Autodesk Inventor part; units mm, degrees
ref_plane "YZ Plane" through (0, 0, 0) normal (1, 0, 0) x (0, 1, 0)
ref_plane "XZ Plane" through (0, 0, 0) normal (0, 1, 0) x (-1, 0, 0)
ref_plane "XY Plane" through (0, 0, 0) normal (0, 0, 1) x (1, 0, 0)
sketch "Sketch1" plane through (0, 0, 0) normal (0, 0, 1) x (1, 0, 0)
  line L0 (-75, 42.5) -> (75, 42.5)
  line L1 (75, 42.5) -> (75, -107.5)
  line L2 (75, -107.5) -> (-75, -107.5)
  line L3 (-75, -107.5) -> (-75, 42.5)
  point P0 (0, 0)
  dimension "d0" = 150
  dimension "d1" = 75
  dimension "d2" = 150
  dimension "d85" = 42.5
extrude "baseExtrusion" add sketch "Sketch1" along normal blind 10
sketch "Sketch3" plane through (0, 0, 10) normal (0, 0, 1) x (1, 0, 0)
  circle A0 centre (0, -22.5) radius 21.25
  line L0 (-75, -107.5) -> (75, -107.5)
  line L1 (-75, 42.5) -> (-75, -107.5)
  line L2 (75, 42.5) -> (-75, 42.5)
  dimension "d16" = 42.5
  dimension "d68" = 75
  dimension "d84" = 65
extrude "objectiveExtrusion" cut sketch "Sketch3" against normal through all
sketch "Sketch5" plane through (0, 0, 10) normal (0, 0, 1) x (1, 0, 0)
  line L0 (30, 15) -> (75, 15)
  line L1 (75, 15) -> (75, 0)
  line L2 (75, 0) -> (30, 0)
  line L3 (22.5, 7.5) -> (22.5, 7.5)
  line L4 (75, -107.5) -> (75, 42.5)
  arc A0 (30, 15) -> (22.5, 7.5) centre (30, 7.5) ccw
  arc A1 (22.5, 7.5) -> (30, 0) centre (30, 7.5) ccw
  circle A2 centre (0, -22.5) radius 21.25
  point P0 (0, 0)
  point P1 (22.5, 15)
  dimension "d34" = 15
  dimension "d35" = 7.5
  dimension "d54" = 30
  dimension "d67" = 30
extrude "cageRodBase1" cut sketch "Sketch5" against normal through all contours L0 L1 L2 A1 A0
mirror "cageRodBase2" about plane through (0, 0, 0) normal (1, 0, 0) of "cageRodBase1"
pattern_linear "cageRodBase34" count 2 spacing 60 along (0, -1, 0) of "cageRodBase1", "cageRodBase2"
sketch "Sketch8" plane through (0, 0, 0) normal (0, 0, -1) x (-1, 0, 0)
  line L0 (75, 0) -> (75, -45)
  line L1 (75, 15) -> (75, 42.5)
  circle A0 centre (0, -22.5) radius 21.25
  point P0 (0, 0)
  point P1 (0, 5)
  point P2 (-23.8157, -36.25)
  point P3 (23.8157, -36.25)
  dimension "d71" = 75
  dimension "d72" = 27.5
  dimension "d75" = 360
hole "objectiveHolderMountingHoles" at (-23.8157, -36.25, 0) at (23.8157, -36.25, 0) at (0, 5, 0) direction (0, 0, 1) diameter 3.242 end through all
sketch "Sketch9" plane through (0, 0, 0) normal (0, 0, -1) x (-1, 0, 0)
  line L0 (75, -60) -> (30, -60)
  line L1 (30, -45) -> (75, -45)
  arc A0 (30, -45) -> (30, -60) centre (30, -52.5) ccw
  point P0 (0, 0)
  point P1 (60, -70)
  point P2 (-60, -70)
  point P3 (60, -22.5)
  point P4 (-60, -22.5)
  point P5 (0, 32.5)
  dimension "d87" = 120
  dimension "d88" = 60
  dimension "d97" = 30
  dimension "d98" = 55
  dimension "d99" = 47.5
hole "m6MountingHoles" at (-60, -70, 0) at (60, -70, 0) at (-60, -22.5, 0) at (60, -22.5, 0) at (0, 32.5, 0) direction (0, 0, 1) diameter 4.917 end through all counterbore diameter 10 counterbore depth 2
sketch "Sketch11" plane through (0, 0, 0) normal (0, 0, -1) x (-1, 0, 0)
  line L0 (31, -107.5) -> (17.5, -107.5)
  line L1 (17.5, -107.5) -> (17.5, -84.25)
  line L2 (24.25, -77.5) -> (24.25, -77.5)
  line L3 (31, -84.25) -> (31, -107.5)
  line L4 (-75, -107.5) -> (75, -107.5)
  arc A0 (31, -84.25) -> (24.25, -77.5) centre (24.25, -84.25) ccw
  arc A1 (24.25, -77.5) -> (17.5, -84.25) centre (24.25, -84.25) ccw
  point P0 (0, 0)
  point P1 (17.5, -77.5)
  dimension "d110" = 13.5
  dimension "d111" = 30
  dimension "d112" = 6.75
  dimension "d113" = 6.75
  dimension "d114" = 24.25
extrude "filterWheelPost1" cut sketch "Sketch11" against normal through all
mirror "filterWheelPost2" about plane through (0, 0, 0) normal (1, 0, 0) of "filterWheelPost1"
equation "\"d68\" = 0.5 * d0"
properties part number "rectangularObjectiveHolder"
For this review, take the finished solid that the model builds, in its own axes (mm). A direction names the side the tool comes from. Give positions to 0.01 mm unless a question says otherwise; leave off trailing zeros. Loops run counter-clockwise (first coordinate to the right, second up) from the corner with the lowest first, then second, coordinate; pieces in that order, holes last. Notation, with made-up numbers: (-16.5, 15) -> (13.5, 15) arc R17 cw to (13.5, 38) -> close; hole circle Ø3 at (-17, 48). An arc over 180 degrees is marked (long way). One line per question, with ' | ' between items.
1) We need section A-A (x = -60). Write out the cut boundary in (y, z).
Resolved:
outline: (-107.5, 0) -> (-75, 0) -> (-75, 2) -> (-72.46, 2) -> (-72.46, 10) -> (-107.5, 10) -> close; (-67.54, 2) -> (-65, 2) -> (-65, 0) -> (-60, 0) -> (-60, 10) -> (-67.54, 10) -> close; (-45, 0) -> (-27.5, 0) -> (-27.5, 2) -> (-24.96, 2) -> (-24.96, 10) -> (-45, 10) -> close; (-20.04, 2) -> (-17.5, 2) -> (-17.5, 0) -> (0, 0) -> (0, 10) -> (-20.04, 10) -> close; (15, 0) -> (42.5, 0) -> (42.5, 10) -> (15, 10) -> close
2) We need section C-C (x = 10.5). Write out the cut boundary in (y, z), plus the area to 3 significant figures.
Resolved:
outline: (-107.5, 0) -> (-40.97, 0) -> (-40.97, 10) -> (-107.5, 10) -> close; (-4.03, 0) -> (42.5, 0) -> (42.5, 10) -> (-4.03, 10) -> close | area: 1,130 mm2
3) To check wall thickness, follow probe 1 along Y at (x, z) = (0, 6.5); probe 2 along Y at (x, z) = (67.5, 7.5); probe 3 along Y at (x, z) = (-60, 0.5). State the ranges of each line that lie inside material, in increasing order.
Resolved:
probe 1: y = -107.5 to -43.75, -1.25 to 3.38, 6.62 to 30.04, 34.96 to 42.5 | probe 2: y = -107.5 to -60, -45 to 0, 15 to 42.5 | probe 3: y = -107.5 to -75, -65 to -60, -45 to -27.5, -17.5 to 0, 15 to 42.5
4) We need section B-B (y = 32.5). Write out the cut boundary in (x, z).
Resolved:
outline: (-75, 0) -> (-5, 0) -> (-5, 2) -> (-2.46, 2) -> (-2.46, 10) -> (-75, 10) -> close; (2.46, 2) -> (5, 2) -> (5, 0) -> (75, 0) -> (75, 10) -> (2.46, 10) -> close
5) Insertion check: pin 1 Ø3 at (x, y) = (-62.5, -24) entering from -Z; pin 2 Ø6 at (y, z) = (-49, 8.5) entering from -X; pin 3 Ø2 at (x, z) = (-20.5, 5) entering from -Y; pin 4 Ø3 at (x, y) = (60, -22.5) entering from -Z. Each pin has a flat end and moves straight along its axis. Give the tip position at first contact, or say it passes through.
Resolved:
pin 1: stops at z = 2 | pin 2: stops at x = -26.26 | pin 3: stops at y = -79.45 | pin 4: passes through
6) The part is to be moulded in two halves that separate along X. For faces 4 (the flat face through (-75, 29, 5)), 5 (the flat face through (-1, -48, 10)), 6 (the flat face through (-17.5, -96, 5)), say which applies: +X half, -X half, draft (parallel to the pull), parting line (faces both ways), or undercut.
Resolved:
face 4: -X half | face 5: draft | face 6: undercut
7) For faces 1 (the flat face through (31, -96, 5)), 2 (the flat face through (61, -25, 2)), 3 (the flat face through (53, 0, 5)), list the 3-axis set-ups (+Z, -Z, +X, -X, +Y, -Y) from which the entire face can be reached by the end or side of a thin tool; tool diameter is ignored.
Resolved:
face 1: +Z, -Z, -Y | face 2: -Z | face 3: +Z, -Z, +X
8) We need section D-D (x = 46). Write out the cut boundary in (y, z).
Resolved:
outline: (-107.5, 0) -> (-60, 0) -> (-60, 10) -> (-107.5, 10) -> close; (-45, 0) -> (0, 0) -> (0, 10) -> (-45, 10) -> close; (15, 0) -> (42.5, 0) -> (42.5, 10) -> (15, 10) -> close
